from build123d import *

# Parameters (mm, degrees)
SKETCH1_R           = 12.5
BOSS_EXTRUDE1_DEPTH = 434.9
SKETCH3_R           = 17.5
BOSS_EXTRUDE3_DEPTH = 10
BOSS_EXTRUDE4_START = 10
SKETCH4_R           = 17.5
BOSS_EXTRUDE4_DEPTH = 10


with BuildPart() as part:
    # Sketch1 → Boss-Extrude1 (new body)
    with BuildSketch(Plane(origin=(0, 0, 0), x_dir=(0, 0, -1), z_dir=(1, 0, 0))):
        Circle(SKETCH1_R)
    extrude(amount=-BOSS_EXTRUDE1_DEPTH)

    # Sketch3 → Boss-Extrude3 (add)
    with BuildSketch(Plane(origin=(0, 0, 0), x_dir=(0, 0, -1), z_dir=(1, 0, 0))):
        Circle(SKETCH3_R)
    extrude(amount=BOSS_EXTRUDE3_DEPTH)

    # Sketch4 → Boss-Extrude4 (add)
    with BuildSketch(Plane.ZY.offset(434.9).offset(BOSS_EXTRUDE4_START)):
        with Locations(Location((0, 0, 0), (0, 0, 180))):
            Circle(SKETCH4_R)
    extrude(amount=-BOSS_EXTRUDE4_DEPTH)


solid = part.part
Can you work these out from the model? Positions are in its coordinate system, mm. A direction names the side the tool comes from. Give positions to 0.01 mm unless a question says otherwise; leave off trailing zeros. Loops run counter-clockwise (first coordinate to the right, second up) from the corner with the lowest first, then second, coordinate; pieces in that order, holes last. Notation, with made-up numbers: (51, 83.25) -> (61, 83.25) arc R14 ccw to (61, 95.25) -> close; hole circle Ø3 at (13.25, 31.25). An arc over 180 degrees is marked (long way). Write item = value, one per line.
1) Suppose I cut it at A-A on y = 0. Write out the boundary of the cut face in (x, z).
Check result:
outline = (-444.9, -17.5) -> (-434.9, -17.5) -> (-434.9, -12.5) -> (0, -12.5) -> (0, -17.5) -> (10, -17.5) -> (10, 17.5) -> (0, 17.5) -> (0, 12.5) -> (-434.9, 12.5) -> (-434.9, 17.5) -> (-444.9, 17.5) -> close
2) Suppose I cut it at C-C on x = -35.5. Write out the boundary of the cut face in (y, z).
Check result:
outline = circle Ø25 at (0, 0)
3) Will these pins go through, and if not, where does the flat tip stop? pin 1 (12 mm diameter, centred on x = -189.5, y = 4.5, fed in from -Z); pin 2 (3 mm diameter, centred on x = -117.5, z = 1.5, fed in from +Y); pin 3 (10 mm diameter, centred on x = -44.5, y = 1.5, fed in from +Z).
Check result:
pin_1 = -12.5
pin_2 = 12.5
pin_3 = 12.5
4) I need wall thicknesses on L1, parallel to X at y = -2.5, z = 15; L2, parallel to Y at x = -19.5, z = 0; L3, parallel to Z at x = -364.5, y = -0.5. Which ranges of each line are inside material? Lowest first, please. Write a range as from..to.
Check result:
L1 = -444.9..-434.9, 0..10
L2 = -12.5..12.5
L3 = -12.49..12.49
5) For faces 4 (the cylindrical face through (4.93, -10.648, 13.887)), 5 (the flat face through (0, -11, -8)), which set-ups out of +Z, -Z, +X, -X, +Y, -Y let a thin tool reach every point of the face, with its end or its side?
Check result:
face_4 = +X, -X
face_5 = none
6) Thinking about a two-plate mould opening in X: for faces 1 (the flat face through (10, 0, 0)), 2 (the cylindrical face through (-214.406, 3.755, -11.923)), 3 (the cylindrical face through (-439.97, 17.084, 3.794)), which applies, released by +X, released by -X, zero draft, split by the parting line, or undercut?
Check result:
face_1 = released by +X
face_2 = undercut
face_3 = zero draft
